from build123d import *

# Parameters (mm, degrees)
F0_W     = 80
F0_H     = 200
F0_R     = 2
F1_DEPTH = 8


with BuildPart() as f1:
    # F0 (on Front) → F1 (new body)
    with BuildSketch(Plane.XZ):
        Rectangle(F0_W, F0_H)
        with Locations((-35.5, -85)):
            Circle(F0_R, mode=Mode.SUBTRACT)
        with Locations((-35.5, -59)):
            Circle(F0_R, mode=Mode.SUBTRACT)
        with Locations((-9.5, -85)):
            Circle(F0_R, mode=Mode.SUBTRACT)
        with Locations((-9.5, -59)):
            Circle(F0_R, mode=Mode.SUBTRACT)
        with Locations((9.5, -85)):
            Circle(F0_R, mode=Mode.SUBTRACT)
        with Locations((9.5, -59)):
            Circle(F0_R, mode=Mode.SUBTRACT)
        with Locations((35.5, -85)):
            Circle(F0_R, mode=Mode.SUBTRACT)
        with Locations((35.5, -59)):
            Circle(F0_R, mode=Mode.SUBTRACT)
        with Locations((-35.5, 59)):
            Circle(F0_R, mode=Mode.SUBTRACT)
        with Locations((-35.5, 85)):
            Circle(F0_R, mode=Mode.SUBTRACT)
        with Locations((-9.5, 59)):
            Circle(F0_R, mode=Mode.SUBTRACT)
        with Locations((-9.5, 85)):
            Circle(F0_R, mode=Mode.SUBTRACT)
        with Locations((9.5, 59)):
            Circle(F0_R, mode=Mode.SUBTRACT)
        with Locations((9.5, 85)):
            Circle(F0_R, mode=Mode.SUBTRACT)
        with Locations((35.5, 59)):
            Circle(F0_R, mode=Mode.SUBTRACT)
        with Locations((35.5, 85)):
            Circle(F0_R, mode=Mode.SUBTRACT)
    extrude(amount=F1_DEPTH)


solid = f1.part
Could you check a few things on this model? Use its own coordinates, in mm. Give positions to 0.01 mm unless a question says otherwise; leave off trailing zeros. Order: outer loops, then holes, each group sorted by start corner. A loop starts at its lowest first (then second) coordinate and runs counter-clockwise, first axis right, second up.
Item 1: I'm going to push a flat-ended pin straight in: pin 1 (3.5 mm diameter, centred on x = 9.5, z = 59, fed in from +Y). Where does the tip first touch, or does it pass through?
Item 2: If we section it at B-B, the plane x = 9.5: Write out the boundary of the cut face in (y, z), plus the area to 3 significant figures.
Item 3: If we section it at A-A, the plane z = 85: Write out the boundary of the cut face in (x, y), plus the area to 3 significant figures.
Item 4: I need wall thicknesses on line 1 (Z direction, x = 35.5, y = -4.75). Which ranges of the line are inside material? Lowest first, please.
Item 5: If we mould it in two halves opening along Z, with no side actions, what happens to faces 1 (the face through (-35.76, -3.944, -57.017)), 2 (the face through (-1, -8, 1)), 3 (the face through (-1, -4, 100))? For each: pulls with the +Z half, pulls with the -Z half, needs draft (parallel to the pull), parting line crosses it, or undercut.
Values:
1. pin 1: passes through
2. outline: (-8, -100) - (0, -100) - (0, -87) - (-8, -87) - close; (-8, -83) - (0, -83) - (0, -61) - (-8, -61) - close; (-8, -57) - (0, -57) - (0, 57) - (-8, 57) - close; (-8, 61) - (0, 61) - (0, 83) - (-8, 83) - close; (-8, 87) - (0, 87) - (0, 100) - (-8, 100) - close
2. area: 1,470 mm2
3. outline: (-40, -8) - (-37.5, -8) - (-37.5, 0) - (-40, 0) - close; (-33.5, -8) - (-11.5, -8) - (-11.5, 0) - (-33.5, 0) - close; (-7.5, -8) - (7.5, -8) - (7.5, 0) - (-7.5, 0) - close; (11.5, -8) - (33.5, -8) - (33.5, 0) - (11.5, 0) - close; (37.5, -8) - (40, -8) - (40, 0) - (37.5, 0) - close
3. area: 512 mm2
4. line 1: z = -100 to -87, -83 to -61, -57 to 57, 61 to 83, 87 to 100
5. face 1: undercut
5. face 2: needs draft
5. face 3: pulls with the +Z half
